Answer from the drawing. Dimensions are ordinates in mm from the lowest x, y and z of the part. A direction names the side the tool comes from. Give positions to 0.01 mm unless a question says otherwise; leave off trailing zeros. Write each loop counter-clockwise with the first axis right and the second up, starting at its lowest first coordinate (ties: lowest second). Pieces come first, ordered by that corner, then holes. Notation, with made-up numbers: M 25.5,88 L 43.5,88 A28 cw 43.5,124 Z; hole C 34.25,49.25 d9. An arc over 180 degrees is marked long. Put each result on its own line as item: value.
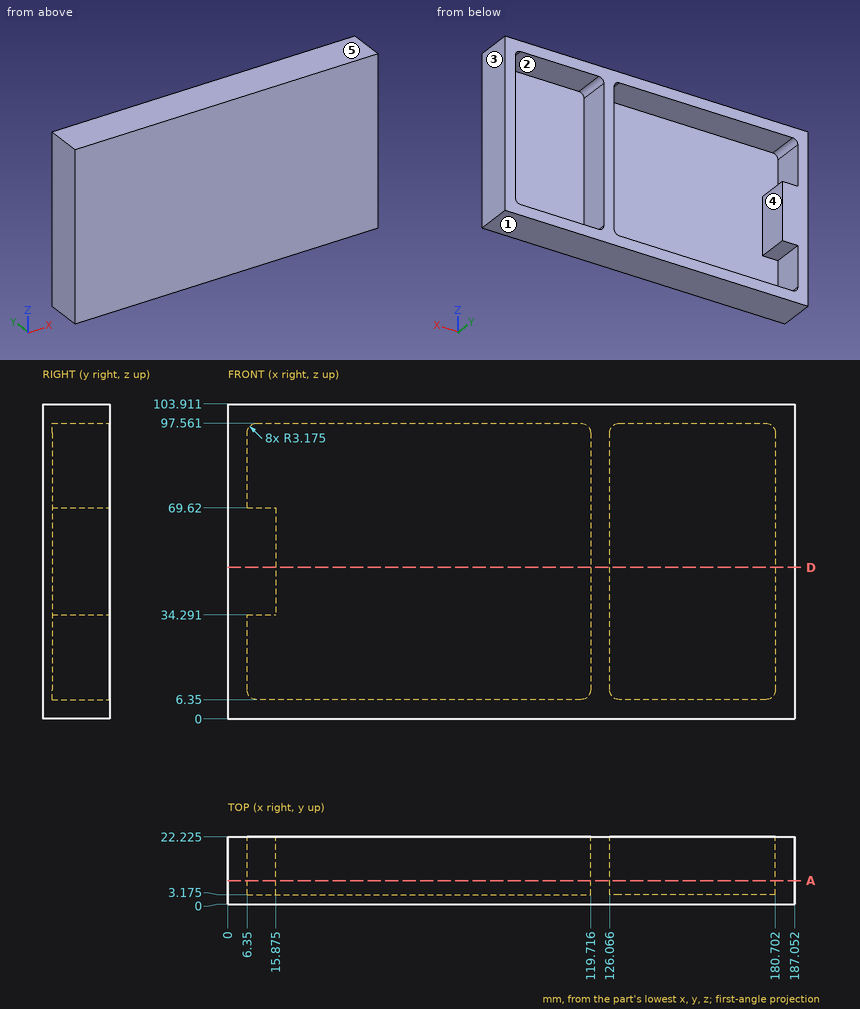
(1) Given pin 1 Ø4 at (x, z) = (25.5, 15.5) entering from +Y (1 decimal), flat-ended and moving along its own axis, determine where the tip first touches the part or whether it passes through.
Result:
pin 1: stops at y = 3.2
(2) Straight lines are drawn through the part: line 1 along X through (y, z) = (15.25, 75.5); line 2 along X through (y, z) = (3.75, 49.5) (1 decimal); line 3 along Z through (x, y) = (148, 15.25). For each, find the intervals that lie inside material, in ascending order. Write a range as from..to.
Result:
line 1: x = 0..6.35, 119.72..126.07, 180.7..187.05
line 2: x = 0..15.9, 119.7..126.1, 180.7..187.1
line 3: z = 0..6.35, 97.56..103.91
(3) Which of the six approach directions +Z, -Z, +X, -X, +Y, -Y give full straight-line access (tool end or side, diameter ignored) to the marked faces 1 and 2?
Result:
face 1: -Z, +X, -X, +Y, -Y
face 2: +Y
(4) Section D-D on z = 50 is taken. Determine the outline of the cut face in (x, y) (1 decimal), and give its area (3 significant figures).
Result:
outline: M 0,0 L 187.1,0 L 187.1,22.2 L 180.7,22.2 L 180.7,3.2 L 126.1,3.2 L 126.1,22.2 L 119.7,22.2 L 119.7,3.2 L 15.9,3.2 L 15.9,22.2 L 0,22.2 Z
area: 1,140 mm²
(5) Section A-A on y = 7.75 is taken. Give the number of separate pieces and of enclosed holes in the cut face, and give its area (3 significant figures).
Result:
separate pieces: 1
enclosed holes: 2
area: 4,470 mm²
(6) For a pull along Z with two mould halves and no side action, classify the marked faces 3, 4 and 5 as +Z half, -Z half, draft (parallel to the pull), parting line (faces both ways), or undercut.
Result:
face 3: draft
face 4: undercut
face 5: +Z half
